Autodesk Inventor part; units mm, degrees
ref_plane "YZ Plane" through (0, 0, 0) normal (1, 0, 0) x (0, 1, 0)
ref_plane "XZ Plane" through (0, 0, 0) normal (0, 1, 0) x (-1, 0, 0)
ref_plane "XY Plane" through (0, 0, 0) normal (0, 0, 1) x (1, 0, 0)
sketch "Sketch1" plane through (0, 0, 0) normal (0, 1, 0) x (-1, 0, 0)
  line L0 (0, 0) -> (25, 0)
  line L1 (25, 0) -> (25, -72)
  line L2 (25, -72) -> (0, -72)
  line L3 (0, -72) -> (0, 0)
  dimension "d0" = 72
  dimension "d1" = 25
extrude "Extrusion1" add sketch "Sketch1" along normal blind 25
sketch "Sketch2" plane through (0, 25, 0) normal (0, 1, 0) x (1, 0, 0)
  line L0 (-21, 5) -> (-4, 5)
  line L1 (-4, 5) -> (-4, 67)
  line L2 (-4, 67) -> (-21, 67)
  line L3 (-21, 67) -> (-21, 5)
  line L4 (-25, 72) -> (-25, 0)
  line L5 (0, 72) -> (-25, 72)
  point P0 (0, 0)
  dimension "d4" = 62
  dimension "d5" = 17
  dimension "d6" = 4
  dimension "d7" = 5
ref_plane "Work Plane1" through (0, 5, 0) normal (0, -1, 0) x (1, 0, 0)
sketch "Sketch3" plane through (0, 5, 0) normal (0, -1, 0) x (1, 0, 0)
  line L0 (-4.5, -55) -> (-20.5, -55)
  line L1 (-20.5, -55) -> (-20.5, -65)
  line L2 (-20.5, -65) -> (-4.5, -65)
  line L3 (-4.5, -65) -> (-4.5, -55)
  line L4 (0, -72) -> (-25, -72)
  line L5 (0, 0) -> (0, -72)
  dimension "d9" = 10
  dimension "d10" = 16
  dimension "d11" = 7
  dimension "d12" = 4.5
loft "Loft1" cut profiles "Sketch2", "Sketch3"
properties part number "Tapered Mould"
Check sheet for the modelled part. Datum: model origin and axes. Units: mm. Round coordinates to 2 decimals unless told otherwise and drop trailing zeros. Write item = value, one per line.
Q1. Go/stop test with flat-tipped pins: pin 1 (1.5 mm diameter, centred on x = -19.5, y = 8.5, fed in from +Z); pin 2 (5 mm diameter, centred on x = -16.5, z = -58.5, fed in from +Y). Record where each tip stops, or that it passes through.
Computed:
pin_1 = 0
pin_2 = 5
Q2. Thickness scan on line 1 along X through (y, z) = (5.25, -57.5); line 2 along X through (y, z) = (18.25, -36.5); line 3 along Y through (x, z) = (-8.5, -57). Record the ranges inside material, lowest first.
Computed:
line_1 = -25 to -20.51, -4.49 to 0
line_2 = -25 to -20.83, -4.17 to 0
line_3 = 0 to 5
Q3. Draft check along X on faces 1 (the face through (-12, 12, 0)), 2 (the face through (-25, 12, -35)), 3 (the face through (-13, 5, -60)). Enter one of: pulls with the +X half, pulls with the -X half, needs draft (parallel to the pull), parting line crosses it, or undercut.
Computed:
face_1 = needs draft
face_2 = pulls with the -X half
face_3 = undercut
